Check sheet for the modelled part. Datum: model origin and axes. Units: mm. Coordinates: 2 decimals unless noted, no trailing zeros. Write each loop counter-clockwise with the first axis right and the second up, starting at its lowest first coordinate (ties: lowest second). Pieces come first, ordered by that corner, then holes. Notation, with made-up numbers: M 20.25,54 L 51.25,54 A32 ccw 51.25,93 Z; hole C 70,7 d10. An arc over 180 degrees is marked long. Answer as CSV lines item,"result". Start each with the question number.
1) Go/stop test with flat-tipped pins: pin 1 Ø0.8 at (x, z) = (220, 3) entering from -Y; pin 2 Ø6 at (x, y) = (272, 7) entering from +Z; pin 3 Ø0.8 at (x, z) = (350, 2.5) entering from +Y. Record where each tip stops, or that it passes through.
2) Section check A-A (z = 2.8). State how many separate pieces and enclosed holes the cut face has, and give its area (3 significant figures).
3) Material ranges on L1, parallel to Z at x = 350, y = 10.25; L2, parallel to Y at x = 185.5, z = 2.3, recorded low to high. Write a range as [from, to].
4) Section check B-B (x = 328.5). Record the cut outline in (y, z), and give its area (3 significant figures).
from build123d import *

# Parameters (mm, degrees)
SKETCH1_W           = 380
SKETCH1_H           = 12
BOSS_EXTRUDE1_DEPTH = 2
SKETCH2_W           = 7
SKETCH2_H           = 7
BOSS_EXTRUDE2_DEPTH = 1.5


with BuildPart() as part:
    # Sketch1 → Boss-Extrude1 (new body)
    with BuildSketch(Plane.XY):
        with Locations((190, 6)):
            Rectangle(SKETCH1_W, SKETCH1_H)
    extrude(amount=BOSS_EXTRUDE1_DEPTH)

    # Sketch2 → Boss-Extrude2 (add)
    with BuildSketch(Plane.XY.offset(2)):
        with Locations((28.5, 6)):
            Rectangle(SKETCH2_W, SKETCH2_H)
        with Locations((60.5, 6)):
            Rectangle(SKETCH2_W, SKETCH2_H)
        with Locations((92.5, 6)):
            Rectangle(SKETCH2_W, SKETCH2_H)
        with Locations((124.5, 6)):
            Rectangle(SKETCH2_W, SKETCH2_H)
        with Locations((156.5, 6)):
            Rectangle(SKETCH2_W, SKETCH2_H)
        with Locations((188.5, 6)):
            Rectangle(SKETCH2_W, SKETCH2_H)
        with Locations((220.5, 6)):
            Rectangle(SKETCH2_W, SKETCH2_H)
        with Locations((252.5, 6)):
            Rectangle(SKETCH2_W, SKETCH2_H)
        with Locations((284.5, 6)):
            Rectangle(SKETCH2_W, SKETCH2_H)
        with Locations((316.5, 6)):
            Rectangle(SKETCH2_W, SKETCH2_H)
        with Locations((348.5, 6)):
            Rectangle(SKETCH2_W, SKETCH2_H)
    extrude(amount=BOSS_EXTRUDE2_DEPTH)


solid = part.part
Results found:
1,pin 1,"stops at y = 2.5"
1,pin 2,"stops at z = 2"
1,pin 3,"stops at y = 9.5"
2,separate pieces,"11"
2,enclosed holes,"0"
2,area,"539 mm2"
3,L1,"z = [0, 2]"
3,L2,"y = [2.5, 9.5]"
4,outline,"M 0,0 L 12,0 L 12,2 L 0,2 Z"
4,area,"24.0 mm2"
